```python
from build123d import *

# Parameters (mm, degrees)
F0_W     = 127
F0_H     = 539.75
F1_DEPTH = 12.7
F2_W     = 12.7
F2_H     = 514.35
F2_H_2   = 12.7
F2_W_2   = 16.901414
F2_W_3   = 84.698586
F2_W_4   = 101.6
F3_DEPTH = 50.8


with BuildPart() as f1:
    # F0 (on Front) → F1 (new body)
    with BuildSketch(Plane.XZ):
        with Locations((27.642982, 223.3254)):
            Rectangle(F0_W, F0_H)
    extrude(amount=F1_DEPTH)

    # F2 (on face) → F3 (join)
    with BuildSketch(Plane(origin=(0, 0, 0), x_dir=(-1, 0, 0), z_dir=(0, 1, 0))):
        with Locations((-84.792982, 223.3254)):
            Rectangle(F2_W, F2_H)
        with Locations((-84.792982, 486.8504)):
            Rectangle(F2_W, F2_H_2)
        with Locations((-69.992275, 486.8504)):
            Rectangle(F2_W_2, F2_H_2)
        with Locations((-19.192275, 486.8504)):
            Rectangle(F2_W_3, F2_H_2)
        with Locations((29.507018, 486.8504)):
            Rectangle(F2_W, F2_H_2)
        with Locations((29.507018, 223.3254)):
            Rectangle(F2_W, F2_H)
        with Locations((29.507018, -40.1996)):
            Rectangle(F2_W, F2_H_2)
        with Locations((-27.642982, -40.1996)):
            Rectangle(F2_W_4, F2_H_2)
        with Locations((-84.792982, -40.1996)):
            Rectangle(F2_W, F2_H_2)
    extrude(amount=F3_DEPTH)


solid = f1.part
```
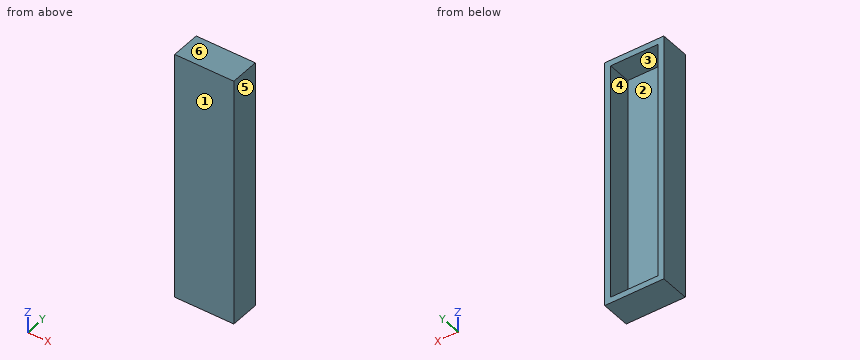
The listing builds one solid part. Answer for the finished solid, in the listing's coordinates (mm). Face numbers are marked on the shaded views. A direction names the side the tool comes from. Round coordinates to 2 decimals unless told otherwise and drop trailing zeros. Write each loop counter-clockwise with the first axis right and the second up, starting at its lowest first coordinate (ties: lowest second). Pieces come first, ordered by that corner, then holes. Notation, with made-up numbers: (-40, 43) -> (-9, 43) arc R28 cw to (-9, 77) -> close; hole circle Ø1 at (-8.75, 68.25). An arc over 180 degrees is marked (long way). Answer as a JSON object with one key per item and string values. Group by question number.
Q1. Which of the six approach directions +Z, -Z, +X, -X, +Y, -Y give full straight-line access (tool end or side, diameter ignored) to the marked faces 1 and 2?
Q2. Section B-B (y = 4.5) is taken. Write down the section's boundary in (x, z).
Q3. Section A-A (x = 23) is taken. Write down the section's boundary in (y, z), plus the area to 3 significant figures.
Q4. Section C-C (z = 223) is taken. Write down the section's boundary in (x, y).
Q5. Straight lines are drawn through the part: line 1 along X through (y, z) = (36, 107); line 2 along Z through (x, y) = (21.5, 25); line 3 along Y through (x, z) = (37, 147). For each, find the intervals that lie inside material, in ascending order.
Q6. This flat-tipped pin is pushed along its axis until it touches: pin 1 Ø8 at (x, z) = (27, 54.5) entering from +Y. Where does it stop, or does it pass through?
Q7. Determine the mould class of the marked faces 3, 4, 5 and 6 for opening direction X: pulls with the +X half, pulls with the -X half, needs draft (parallel to the pull), parting line crosses it, or undercut.
Check values:
{
 "1": {"face 1": "+Z, -Z, +X, -X, -Y", "face 2": "+Y"},
 "2": {"outline": "(-35.86, -46.55) -> (91.14, -46.55) -> (91.14, 493.2) -> (-35.86, 493.2) -> close; hole (-23.16, -33.85) -> (78.44, -33.85) -> (78.44, 480.5) -> (-23.16, 480.5) -> close"},
 "3": {"outline": "(-12.7, -46.55) -> (50.8, -46.55) -> (50.8, -33.85) -> (0, -33.85) -> (0, 480.5) -> (50.8, 480.5) -> (50.8, 493.2) -> (-12.7, 493.2) -> close", "area": "8,150 mm^2"},
 "4": {"outline": "(-35.86, -12.7) -> (91.14, -12.7) -> (91.14, 50.8) -> (78.44, 50.8) -> (78.44, 0) -> (-23.16, 0) -> (-23.16, 50.8) -> (-35.86, 50.8) -> close"},
 "5": {"line 1": "-35.86 to -23.16, 78.44 to 91.14", "line 2": "-46.55 to -33.85, 480.5 to 493.2", "line 3": "-12.7 to 0"},
 "6": {"pin 1": "y = 0"},
 "7": {"face 3": "undercut", "face 4": "undercut", "face 5": "pulls with the +X half", "face 6": "needs draft"}
}
